Could you check a few things on this model? Use its own coordinates, in mm. Face numbers are marked on the shaded views. A direction names the side the tool comes from. Round coordinates to 2 decimals unless told otherwise and drop trailing zeros. Order: outer loops, then holes, each group sorted by start corner. A loop starts at its lowest first (then second) coordinate and runs counter-clockwise, first axis right, second up. Notation, with made-up numbers: M 85.25,-25.75 L 90.25,-25.75 A27 cw 90.25,1.25 Z; hole C -4,19 d4. An arc over 180 degrees is marked long. Write each question's results on one line, items separated by ' | '. Start each with the question number.
1. Suppose I cut it at D-D on y = -32. Write out the boundary of the cut face in (x, z), and give its area (3 significant figures).
2. Please list where these lines run through material, in increasing order: L1, parallel to X at y = -40.5, z = 146.75; L2, parallel to X at y = -43.5, z = 151.25; L3, parallel to Y at x = -10, z = 143.
3. Suppose I cut it at C-C on z = 151. Write out the boundary of the cut face in (x, y).
4. Suppose I cut it at B-B on x = -7.25. Write out the boundary of the cut face in (y, z), and give its area (3 significant figures).
5. I'm going to push flat-ended pins straight in: pin 1 (6 mm diameter, centred on x = -5, z = 132, fed in from +Y); pin 2 (1.5 mm diameter, centred on x = -2, z = 151, fed in from +Y); pin 3 (3 mm diameter, centred on x = -2.5, y = -42.5, fed in from -Z). Where does each tip first touch, or does it pass through?
6. We'd pull the mould along Z, two halves only. Please class the marked faces 1, 2 and 3: released by +Z, released by -Z, zero draft, split by the parting line, or undercut.
7. Suppose I cut it at A-A on y = -45.75. Write out the boundary of the cut face in (x, z), and give its area (3 significant figures).
8. For the marked faces 4, 5, 6 and 7, which set-ups out of +Z, -Z, +X, -X, +Y, -Y let a thin tool reach every point of the face, with its end or its side?
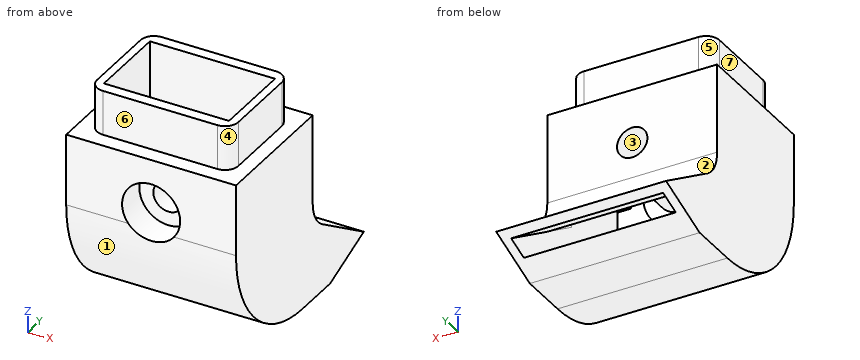
from build123d import *

# Parameters (mm, degrees)
SALIENTE_EXTRUIR1_DEPTH                              = 18
SALIENTE_EXTRUIR2_DEPTH                              = 12
CORTAR_EXTRUIR1_DEPTH                                = 17
CROQUIS4_W                                           = 16.47485784
CROQUIS4_H                                           = 9
CORTAR_EXTRUIR2_DEPTH                                = 15.5
CORTAR_EXTRUIR3_DEPTH                                = 5
CROQUIS6_W                                           = 18
CROQUIS6_H                                           = 12.211968345
CORTAR_EXTRUIR4_DEPTH                                = 27.564918354
SALIENTE_EXTRUIR3_DEPTH                              = 9
SALIENTE_EXTRUIR4_DEPTH                              = 1.25
CROQUIS9_W                                           = 18
CROQUIS9_H                                           = 21
SALIENTE_EXTRUIR5_DEPTH                              = 1.75
CROQUIS10_W                                          = 1.5
CROQUIS10_H                                          = 9
CORTAR_EXTRUIR5_DEPTH                                = 6.47485784
CROQUIS11_W                                          = 1.5
CROQUIS11_H                                          = 9
CORTAR_EXTRUIR6_DEPTH                                = 6.47485784
SALIENTE_EXTRUIR6_DEPTH                              = 1
NGULO_DE_SALIDA1_ANGLE                               = 32.6
REFRENTADO_PARA_TORNILLO_CON_CABEZA_HEXA_D           = 3.4
REFRENTADO_PARA_TORNILLO_CON_CABEZA_HEXA_DEPTH       = 24.997848167
REFRENTADO_PARA_TORNILLO_CON_CABEZA_HEXA_CBORE_D     = 6.5
REFRENTADO_PARA_TORNILLO_CON_CABEZA_HEXA_CBORE_DEPTH = 3.4
REDONDEO1_R                                          = 1.5
REDONDEO2_R                                          = 4.046592592
REDONDEO3_R                                          = 9.394473
REDONDEO4_R                                          = 10
REDONDEO5_R                                          = 13.000000028


with BuildPart() as part:
    # Croquis1 → Saliente-Extruir1 (new body)
    with BuildSketch(Plane(origin=(7.936078108, 0, 0), x_dir=(0, 0, -1), z_dir=(1, 0, 0))):
        with BuildLine():
            Line((-154.285744598, -37.213626554), (-128.285744598, -37.213626554))
            Line((-128.285744598, -37.213626554), (-128.285744598, -33.793626733))
            Line((-128.285744598, -33.793626733), (-137.073776253, -9.6487082))
            Line((-137.073776253, -9.6487082), (-149.285744598, -9.6487082))
            add(Edge.make_bspline(
                [(-154.285744598, -9.6487082), (-152.619077931, -9.6487082), (-150.952411265, -9.6487082), (-149.285744598, -9.6487082)],
                knots=[0, 0, 0, 0, 1, 1, 1, 1], degree=3))
            add(Edge.make_bspline(
                [(-154.285744598, -9.6487082), (-154.285744598, -18.837014318), (-154.285744598, -28.025320436), (-154.285744598, -37.213626554)],
                knots=[0, 0, 0, 0, 1, 1, 1, 1], degree=3))
        make_face()
    extrude(amount=-SALIENTE_EXTRUIR1_DEPTH)

    # Croquis2 → Saliente-Extruir2 (add)
    with BuildSketch(Plane.XZ.offset(37.213626554)):
        with BuildLine():
            Line((-10.063921892, 154.285744598), (7.936078108, 154.285744598))
            add(Edge.make_bspline(
                [(7.936078108, 154.285744598), (7.936078108, 152.619077931), (7.936078108, 150.952411265), (7.936078108, 149.285744598)],
                knots=[0, 0, 0, 0, 1, 1, 1, 1], degree=3))
            Line((7.936078108, 149.285744598), (7.936078108, 128.285744598))
            Line((7.936078108, 128.285744598), (-10.063921892, 128.285744598))
            Line((-10.063921892, 128.285744598), (-10.063921892, 154.285744598))
        make_face()
    extrude(amount=SALIENTE_EXTRUIR2_DEPTH)

    # Croquis3 → Cortar-Extruir1 (cut)
    with BuildSketch(Plane.ZY.offset(10.063921892)):
        Polygon((135.078487354, -49.213626554), (137.810886758, -49.213626554), (137.810886758, -40.213626554), (130.25136436, -28.393130822), (129.348598898, -30.873458543), align=None)
    extrude(amount=-CORTAR_EXTRUIR1_DEPTH, mode=Mode.SUBTRACT)

    # Croquis4 → Cortar-Extruir2 (cut)
    with BuildSketch(Plane.ZY.offset(10.063921892)):
        with Locations((146.048315678, -44.713626554)):
            Rectangle(CROQUIS4_W, CROQUIS4_H)
    extrude(amount=-CORTAR_EXTRUIR2_DEPTH, mode=Mode.SUBTRACT)

    # Croquis5 → Cortar-Extruir3 (cut)
    with BuildSketch(Plane.XY.offset(154.285744598)):
        with BuildLine():
            Line((-10.063921892, -40.213626554), (-9.463921892, -40.213626554))
            Line((-9.463921892, -40.213626554), (-9.463921892, -38.963626554))
            Line((-9.463921892, -38.963626554), (6.336078108, -38.963626554))
            Line((6.336078108, -38.963626554), (6.336078108, -49.213626554))
            Line((6.336078108, -49.213626554), (7.936078108, -49.213626554))
            Line((7.936078108, -49.213626554), (7.936078108, -37.213626554))
            add(Edge.make_bspline(
                [(7.936078108, -9.6487082), (7.936078108, -18.837014318), (7.936078108, -28.025320436), (7.936078108, -37.213626554)],
                knots=[0, 0, 0, 0, 1, 1, 1, 1], degree=3))
            Line((7.936078108, -9.6487082), (-10.063921892, -9.6487082))
            add(Edge.make_bspline(
                [(-10.063921892, -9.6487082), (-10.063921892, -18.837014318), (-10.063921892, -28.025320436), (-10.063921892, -37.213626554)],
                knots=[0, 0, 0, 0, 1, 1, 1, 1], degree=3))
            Line((-10.063921892, -37.213626554), (-10.063921892, -40.213626554))
        make_face()
    extrude(amount=-CORTAR_EXTRUIR3_DEPTH, mode=Mode.SUBTRACT)

    # Croquis6 → Cortar-Extruir4 (cut)
    with BuildSketch(Plane(origin=(0, -9.6487082, 0), x_dir=(-1, 0, 0), z_dir=(0, 1, 0))):
        with Locations((1.063921892, 143.179760426)):
            Rectangle(CROQUIS6_W, CROQUIS6_H)
    extrude(amount=-CORTAR_EXTRUIR4_DEPTH, mode=Mode.SUBTRACT)

    # Croquis7 → Saliente-Extruir3 (add)
    with BuildSketch(Plane.XZ.offset(40.213626554)):
        Polygon((-9.463921892, 154.285744598), (-8.563921892, 154.285744598), (-8.563921892, 137.810886758), (-10.063921892, 137.810886758), (-10.063921892, 149.285744598), (-9.463921892, 149.285744598), align=None)
    extrude(amount=SALIENTE_EXTRUIR3_DEPTH)

    # Croquis8 → Saliente-Extruir4 (add)
    with BuildSketch(Plane.XZ.offset(49.213626554)):
        Polygon((-9.463921892, 154.285744598), (6.336078108, 154.285744598), (6.336078108, 149.285744598), (7.936078108, 149.285744598), (7.936078108, 128.285744598), (-10.063921892, 128.285744598), (-10.063921892, 149.285744598), (-9.463921892, 149.285744598), align=None)
    extrude(amount=SALIENTE_EXTRUIR4_DEPTH)

    # Croquis9 → Saliente-Extruir5 (add)
    with BuildSketch(Plane.XZ.offset(50.463626554)):
        with Locations((-1.063921892, 138.785744598)):
            Rectangle(CROQUIS9_W, CROQUIS9_H)
    extrude(amount=SALIENTE_EXTRUIR5_DEPTH)

    # Croquis10 → Cortar-Extruir5 (cut)
    with BuildSketch(Plane(origin=(0, 0, 137.810886758), x_dir=(-1, 0, 0), z_dir=(0, 0, -1))):
        with Locations((-6.186078108, -44.713626554)):
            Rectangle(CROQUIS10_W, CROQUIS10_H)
    extrude(amount=-CORTAR_EXTRUIR5_DEPTH, mode=Mode.SUBTRACT)

    # Croquis11 → Cortar-Extruir6 (cut)
    with BuildSketch(Plane(origin=(0, 0, 137.810886758), x_dir=(-1, 0, 0), z_dir=(0, 0, -1))):
        with Locations((9.313921892, -44.713626554)):
            Rectangle(CROQUIS11_W, CROQUIS11_H)
    extrude(amount=-CORTAR_EXTRUIR6_DEPTH, mode=Mode.SUBTRACT)

    # Croquis12 → Saliente-Extruir6 (add)
    with BuildSketch(Plane.ZY.offset(10.063921892)):
        Polygon((149.285744598, -52.213626554), (128.285744598, -52.213626554), (128.285744598, -33.793626733), (137.073776253, -9.6487082), (137.073776253, -37.213626554), (149.285744598, -37.213626554), align=None)
    extrude(amount=SALIENTE_EXTRUIR6_DEPTH)

    # Ángulo de salida1
    ngulo_de_salida1_faces = [part.faces().sort_by_distance(p)[0] for p in [
        (-1.563921892, -23.431167377, 137.073776253),
    ]]
    draft(ngulo_de_salida1_faces, Plane.ZX.offset(-37.213626554), NGULO_DE_SALIDA1_ANGLE)

    # Croquis13 → Revolución1 (revolve)
    with BuildSketch(Plane(origin=(0, 0, 143.285744598), x_dir=(-1, 0, 0), z_dir=(0, 0, -1)), mode=Mode.PRIVATE) as revoluci_n1_sk:
        Polygon((-2.686078108, -49.213626554), (1.563921892, -49.213626554), (1.563921892, -40.213626554), (-1.136078108, -40.213626554), (-1.136078108, -46.813626554), (-2.686078108, -46.813626554), align=None)
    revolve(revoluci_n1_sk.sketch.rotate(Axis((-1.563921892, -49.213626554, 143.285744598), (0, 1, 0)), 270), axis=Axis((-1.563921892, -49.213626554, 143.285744598), (0, 1, 0)))

    # Refrentado para tornillo con cabeza hexagonal de M31
    with Locations(Plane(origin=(0, -52.213626554, 0), x_dir=(-1, 0, 0), z_dir=(0, -1, 0))):
        with Locations((1.563921892, -143.285744598)):
            CounterBoreHole(REFRENTADO_PARA_TORNILLO_CON_CABEZA_HEXA_D / 2, REFRENTADO_PARA_TORNILLO_CON_CABEZA_HEXA_CBORE_D / 2, REFRENTADO_PARA_TORNILLO_CON_CABEZA_HEXA_CBORE_DEPTH, depth=REFRENTADO_PARA_TORNILLO_CON_CABEZA_HEXA_DEPTH)

    # Redondeo1
    redondeo1_edges = [part.edges().sort_by_distance(p)[0] for p in [
        (6.336078108, -50.463626554, 151.785744598),
        (6.336078108, -38.963626554, 151.785744598),
        (-9.463921892, -50.463626554, 151.785744598),
        (-9.463921892, -38.963626554, 151.785744598),
    ]]
    fillet(redondeo1_edges, radius=REDONDEO1_R)

    # Redondeo2
    redondeo2_edges = [part.edges().sort_by_distance(p)[0] for p in [
        (-1.563921892, -37.213626554, 137.073776253),
    ]]
    fillet(redondeo2_edges, radius=REDONDEO2_R)

    # Redondeo3
    # the kernel refuses this fillet: 9.394473 mm, written as the material it adds along each edge
    with BuildSketch(Plane(origin=(-10.063921892, -49.213626554, 135.078487354), x_dir=(0, 0.954500927456638, -0.2982079467157403), z_dir=(1, 0, 0))) as redondeo3_piece_1_section:
        with BuildLine():
            CenterArc((REDONDEO3_R * 0.735245019776, REDONDEO3_R), REDONDEO3_R, 197.35, 72.65)
            Line((-REDONDEO3_R * 0.21925590768, REDONDEO3_R * 0.701792053284), (0, 0))
            Line((0, 0), (REDONDEO3_R * 0.735245019776, 0))
        make_face()
    redondeo3_piece_1 = extrude(amount=17, mode=Mode.PRIVATE)
    redondeo3_piece_1 = redondeo3_piece_1 - Plane(origin=(-1.563921892, -47.780974958, 143.285744598), x_dir=(0, 0, 1), z_dir=(0, -1, 0)) * Cylinder(4.25, 62, mode=Mode.PRIVATE)
    add(redondeo3_piece_1)

    # Redondeo4
    # the kernel refuses this fillet: 10 mm, written as the material it takes off along each edge
    with BuildSketch(Plane(origin=(6.936078108, -40.213626554, 137.810886758), x_dir=(-2.541450920679997e-12, 0, 1.0), z_dir=(-1.0, -2.5749151914609573e-12, -2.5414509206799975e-12))) as redondeo4_piece_1_section:
        with BuildLine():
            CenterArc((REDONDEO4_R * 0.547484008153, REDONDEO4_R), REDONDEO4_R, 212.6, 57.4)
            Line((-REDONDEO4_R * 0.294968388853, REDONDEO4_R * 0.461229214991), (0, 0))
            Line((0, 0), (REDONDEO4_R * 0.547484008153, 0))
        make_face()
    redondeo4_piece_1 = extrude(amount=15.5, mode=Mode.PRIVATE)
    redondeo4_piece_1 = redondeo4_piece_1 - Plane(origin=(-1.563921892, -39.236985305, 143.285744598), x_dir=(0, 0, 1), z_dir=(0, -1, 0)) * Cylinder(2.7, 53, mode=Mode.PRIVATE)
    add(redondeo4_piece_1, mode=Mode.SUBTRACT)
    with BuildSketch(Plane(origin=(-10.063921892, -40.213626554, 137.810886758), x_dir=(0, 0, 1), z_dir=(1, 0, 0))) as redondeo4_piece_2:
        with BuildLine():
            CenterArc((REDONDEO4_R * 0.547484008153, -REDONDEO4_R), REDONDEO4_R, 90, 57.4)
            Line((-REDONDEO4_R * 0.294968388853, -REDONDEO4_R * 0.461229214991), (0, 0))
            Line((0, 0), (REDONDEO4_R * 0.547484008153, 0))
        make_face()
    extrude(amount=1.5, mode=Mode.SUBTRACT)

    # Redondeo5
    # the kernel refuses this fillet: 13.000000028 mm, written as the material it takes off along each edge
    with BuildSketch(Plane(origin=(40.436078177, -52.213626554, 128.285744598), x_dir=(0, 1, 0), z_dir=(-1, 0, 0))) as redondeo5_piece_1:
        with BuildLine():
            CenterArc((REDONDEO5_R, -REDONDEO5_R), REDONDEO5_R, 90, 90)
            Line((0, -REDONDEO5_R), (0, 0))
            Line((0, 0), (REDONDEO5_R, 0))
        make_face()
    extrude(amount=84.000000138, mode=Mode.SUBTRACT)


solid = part.part
Filled sheet:
1) outline: M -11.06,128.94 L 7.94,128.94 L 7.94,133.74 L -11.06,133.74 Z; hole M -10.06,129.7 L 6.94,129.7 L 6.94,132.56 L -10.06,132.56 Z | area: 42.6 mm^2
2) L1: x = -11.06 to -8.56, 5.44 to 7.94 | L2: x = -9.46 to -8.56, 5.44 to 6.34 | L3: y = -52.21 to -49.21, -40.21 to -37.21
3) outline: M -9.46,-48.96 A1.5 ccw -7.96,-50.46 L 4.84,-50.46 A1.5 ccw 6.34,-48.96 L 6.34,-40.46 A1.5 ccw 4.84,-38.96 L -7.96,-38.96 A1.5 ccw -9.46,-40.46 Z; hole M -8.56,-49.21 L 5.44,-49.21 L 5.44,-40.21 L -8.56,-40.21 Z
4) outline: M -52.21,141.29 A13 ccw -39.21,128.29 L -33.79,128.29 L -30.87,129.35 L -42.62,133.02 A9.39 cw -49.21,141.99 L -49.21,154.29 L -50.46,154.29 L -50.46,149.29 L -52.21,149.29 Z; M -40.21,143.29 A10 ccw -35.6,134.86 L -28.39,130.25 L -27.22,130.68 L -35.35,135.88 A4.05 cw -37.21,139.29 L -37.21,149.29 L -38.96,149.29 L -38.96,154.29 L -40.21,154.29 Z | area: 163 mm^2
5) pin 1: stops at y = -27.22 | pin 2: stops at y = -38.96 | pin 3: stops at z = 128.41
6) face 1: released by -Z | face 2: released by +Z | face 3: undercut
7) outline: M -11.06,130.05 L 7.94,130.05 L 7.94,149.29 L 6.34,149.29 L 6.34,154.29 L 5.44,154.29 L 5.44,144.29 L 6.94,144.29 L 6.94,134.7 L -10.06,134.7 L -10.06,144.29 L -8.56,144.29 L -8.56,154.29 L -9.46,154.29 L -9.46,149.29 L -11.06,149.29 Z; C -1.56,143.29 d5.4; hole C -1.56,143.29 d3.4 | area: 155 mm^2
8) face 4: +Z, +X, -Y | face 5: +Z, -X, +Y | face 6: +Z, +X, -X, -Y | face 7: +Z, -X, +Y, -Y
